CAD build for the part. Positions are in the model's coordinates, mm. A direction names the side the tool comes from. Round coordinates to 2 decimals unless told otherwise and drop trailing zeros. Order: outer loops, then holes, each group sorted by start corner. A loop starts at its lowest first (then second) coordinate and runs counter-clockwise, first axis right, second up. Notation, with made-up numbers: (64, 71) -> (76, 71) arc R23 cw to (76, 83) -> close; hole circle Ø11 at (-2.5, 73). An arc over 180 degrees is marked (long way). Return JSON: item names as keys, results as strings. Group by question number.
Q1. Probe line 1 along X through (y, z) = (-26.5, 5.25); line 2 along X through (y, z) = (25, 7.75); line 3 along X through (y, z) = (23, 8.5). List the from-to ranges inside material, lowest first.
Q2. Cut at D-D (z = 2.25). Count the separate pieces of the cut face and the enclosed holes in it, then the cut area to 3 significant figures.
Q3. Cut at C-C (y = -19). Write the cut outline in (x, z), then the cut area to 3 significant figures.
Q4. Mould opens along X. For faces 4 (the flat face through (2.4, 2.4, 0)), 5 (the flat face through (14.54, 11.71, 4.93)), 6 (the cylindrical face through (-21.89, -25.04, 5.07)) say: +X half, -X half, draft (parallel to the pull), parting line (faces both ways), or undercut.
Q5. Which spindle directions (+Z, -Z, +X, -X, +Y, -Y) get a long thin tool onto all of the face, cutting with end or side? Do faces 1 (the cylindrical face through (25.07, 21.9, 5.07)), 2 (the flat face through (-14.81, 11.98, 4.93)), 3 (the flat face through (-11.71, 14.54, 4.93)). Say none if no direction does.
Q6. Cut at B-B (x = -8). Write the cut outline in (y, z).
Q7. Flat gauge pins, fed straight in: pin 1 (1 mm diameter, centred on y = -2, z = 8.5, fed in from +X); pin 2 (4 mm diameter, centred on y = -21.5, z = 5, fed in from +X); pin 3 (1.5 mm diameter, centred on y = -12, z = 5.5, fed in from -X). Where does each tip first touch, or does it go through?
Q8. Cut at A-A (x = -25). Write the cut outline in (y, z), then the cut area to 3 significant figures.
from build123d import *

# Parameters (mm, degrees)
BOSS_EXTRUDE1_DEPTH = 10
CIRPATTERN1_COUNT   = 4
FILLET1_R           = 2.5


with BuildPart() as part:
    # Sketch1 → Boss-Extrude1 (new body)
    with BuildSketch(Plane.XY):
        with BuildLine():
            ThreePointArc((-25.080279294, 22.251852169), (-23.334523779, 23.334523779), (-22.251852169, 25.080279294))
            Line((-22.251852169, 25.080279294), (-24.04163056, 26.870057685))
            ThreePointArc((-24.04163056, 26.870057685), (-24.022793772, 26.693726845), (-24.016504294, 26.516504294))
            ThreePointArc((-24.016504294, 26.516504294), (-24.878499941, 24.627869407), (-26.870057685, 24.04163056))
            Line((-26.870057685, 24.04163056), (-25.080279294, 22.251852169))
        make_face()
        with BuildLine():
            Line((-24.04163056, 26.870057685), (-22.251852169, 25.080279294))
            ThreePointArc((-22.251852169, 25.080279294), (-22.075731019, 25.788814307), (-22.016504294, 26.516504294))
            ThreePointArc((-22.016504294, 26.516504294), (-30.171159716, 29.142050666), (-25.080279294, 22.251852169))
            Line((-25.080279294, 22.251852169), (-26.870057685, 24.04163056))
            ThreePointArc((-26.870057685, 24.04163056), (-28.284271247, 28.284271247), (-24.04163056, 26.870057685))
        make_face()
        with BuildLine():
            ThreePointArc((-4.264652125, 1.436225), (-3.181980515, 3.181980515), (-1.436225, 4.264652125))
            Line((-1.436225, 4.264652125), (-22.251852169, 25.080279294))
            ThreePointArc((-22.251852169, 25.080279294), (-23.334523779, 23.334523779), (-25.080279294, 22.251852169))
            Line((-25.080279294, 22.251852169), (-4.264652125, 1.436225))
        make_face()
        with BuildLine():
            ThreePointArc((-2.995352392, 0.166925268), (-2.121320344, 2.121320344), (-0.166925268, 2.995352392))
            Line((-0.166925268, 2.995352392), (-1.436225, 4.264652125))
            ThreePointArc((-1.436225, 4.264652125), (-3.181980515, 3.181980515), (-4.264652125, 1.436225))
            Line((-4.264652125, 1.436225), (-2.995352392, 0.166925268))
        make_face()
        with BuildLine():
            Line((-1.436225, 4.264652125), (-0.166925268, 2.995352392))
            ThreePointArc((-0.166925268, 2.995352392), (2.061458731, 2.179538461), (3, 0))
            ThreePointArc((3, 0), (-0.083494978, -2.998837873), (-2.995352392, 0.166925268))
            Line((-2.995352392, 0.166925268), (-4.264652125, 1.436225))
            ThreePointArc((-4.264652125, 1.436225), (-0.727689988, -4.440773275), (4.5, 0))
            ThreePointArc((4.5, 0), (2.625546372, 3.654655422), (-1.436225, 4.264652125))
        make_face()
    extrude(amount=BOSS_EXTRUDE1_DEPTH)


with BuildPart() as cirpattern1_1:
    # CirPattern1: pattern copy
    add(part.part.rotate(Axis((0, 0, 0), (0, 0, 1)), 1 * 360 / CIRPATTERN1_COUNT))


with BuildPart() as cirpattern1_2:
    # CirPattern1: pattern copy
    add(part.part.rotate(Axis((0, 0, 0), (0, 0, 1)), 2 * 360 / CIRPATTERN1_COUNT))


with BuildPart() as cirpattern1_3:
    # CirPattern1: pattern copy
    add(part.part.rotate(Axis((0, 0, 0), (0, 0, 1)), 3 * 360 / CIRPATTERN1_COUNT))

    # Combine1: read off the stored shape, not the designer's step
    # Combine1: union CirPattern1_2, CirPattern1_1, part
    add(cirpattern1_2.part)
    add(cirpattern1_1.part)
    add(part.part)

    # Fillet1
    fillet1_edges = [cirpattern1_3.edges().sort_by_distance(p)[0] for p in [
        (-4.264652125, 1.436225, 5),
        (-25.080279294, 22.251852169, 5),
        (-22.251852169, 25.080279294, 5),
        (-1.436225, 4.264652125, 5),
        (-1.436225, -4.264652125, 5),
        (1.436225, 4.264652125, 5),
        (4.264652125, -1.436225, 5),
        (4.264652125, 1.436225, 5),
        (25.080279294, 22.251852169, 5),
        (22.251852169, 25.080279294, 5),
        (22.251852169, -25.080279294, 5),
        (25.080279294, -22.251852169, 5),
        (1.436225, -4.264652125, 5),
        (-4.264652125, -1.436225, 5),
        (-25.080279294, -22.251852169, 5),
        (-22.251852169, -25.080279294, 5),
    ]]
    fillet(fillet1_edges, radius=FILLET1_R)


solid = cirpattern1_3.part
Solution:
{
 "1": {"line 1": "x = -31.02 to -29.02, -24.02 to -22.02, 22.02 to 24.02, 29.02 to 31.02", "line 2": "x = -30.75 to -28.5, -24.53 to -21.87, 21.87 to 24.53, 28.5 to 30.75", "line 3": "x = -29.32 to -20.17, 20.17 to 29.32"},
 "2": {"separate pieces": "1", "enclosed holes": "5", "area": "676 mm²"},
 "3": {"outline": "(-21.83, 0) -> (-16.17, 0) -> (-16.17, 10) -> (-21.83, 10) -> close; (16.17, 0) -> (21.83, 0) -> (21.83, 10) -> (16.17, 10) -> close", "area": "113 mm²"},
 "4": {"face 4": "draft", "face 5": "+X half", "face 6": "undercut"},
 "5": {"face 1": "+Z, -Z", "face 2": "+Z, -Z, -X", "face 3": "+Z, -Z, +Y"},
 "6": {"outline": "(-10.83, 0) -> (-5.17, 0) -> (-5.17, 10) -> (-10.83, 10) -> close; (5.17, 0) -> (10.83, 0) -> (10.83, 10) -> (5.17, 10) -> close"},
 "7": {"pin 1": "stops at x = 5.33", "pin 2": "stops at x = 29.86", "pin 3": "stops at x = -15.58"},
 "8": {"outline": "(-30.75, 0) -> (-28.5, 0) -> (-28.5, 10) -> (-30.75, 10) -> close; (-24.53, 0) -> (-21.87, 0) -> (-21.87, 10) -> (-24.53, 10) -> close; (21.87, 0) -> (24.53, 0) -> (24.53, 10) -> (21.87, 10) -> close; (28.5, 0) -> (30.75, 0) -> (30.75, 10) -> (28.5, 10) -> close", "area": "98.1 mm²"}
}
